Geometry: final body of the model. Coordinates: model frame, mm. A direction names the side the tool comes from. Round coordinates to 2 decimals unless told otherwise and drop trailing zeros. Loops run counter-clockwise (first coordinate to the right, second up) from the corner with the lowest first, then second, coordinate; pieces in that order, holes last. Notation, with made-up numbers: (-8.5, 80) - (37.5, 80) arc R8 cw to (37.5, 84) - close; hole circle Ø11 at (-35, -11.75). An arc over 180 degrees is marked (long way). Answer as CSV lines item,"result".
from build123d import *

# Parameters (mm, degrees)
SKETCH1_R           = 25.5
BOSS_EXTRUDE1_DEPTH = 4
SKETCH2_R           = 24.5
SKETCH2_R_2         = 18.5
CUT_EXTRUDE1_DEPTH  = 1.675
FILLET1_R           = 1.5
SKETCH3_R           = 14
CUT_EXTRUDE2_DEPTH  = 4
FILLET2_R           = 2
SKETCH4_R           = 1.25
CUT_EXTRUDE3_DEPTH  = 17
SKETCH5_R           = 1.25
CUT_EXTRUDE5_DEPTH  = 17


with BuildPart() as part:
    # Sketch1 → Boss-Extrude1 (new body)
    with BuildSketch(Plane.XY):
        Circle(SKETCH1_R)
    extrude(amount=BOSS_EXTRUDE1_DEPTH)

    # Sketch2 → Cut-Extrude1 (cut)
    with BuildSketch(Plane.XY.offset(4)):
        Circle(SKETCH2_R)
        Circle(SKETCH2_R_2, mode=Mode.SUBTRACT)
    extrude(amount=-CUT_EXTRUDE1_DEPTH, mode=Mode.SUBTRACT)

    # Fillet1
    fillet1_edges = [part.edges().sort_by_distance(p)[0] for p in [
        (-24.5, 0, 2.325),
        (-18.5, 0, 2.325),
    ]]
    fillet(fillet1_edges, radius=FILLET1_R)

    # Sketch3 → Cut-Extrude2 (cut)
    with BuildSketch(Plane.XY.offset(4)):
        Circle(SKETCH3_R)
    extrude(amount=-CUT_EXTRUDE2_DEPTH, mode=Mode.SUBTRACT)

    # Fillet2
    fillet2_edges = [part.edges().sort_by_distance(p)[0] for p in [
        (-25.5, 0, 0),
    ]]
    fillet(fillet2_edges, radius=FILLET2_R)

    # Sketch4 → Cut-Extrude3 (cut)
    with BuildSketch(Plane(origin=(0, 0, 0), x_dir=(0, 0, -1), z_dir=(1, 0, 0))):
        with Locations((-2, 0)):
            Circle(SKETCH4_R)
    extrude(amount=-CUT_EXTRUDE3_DEPTH, mode=Mode.SUBTRACT)

    # Sketch5 → Cut-Extrude5 (cut, symmetric)
    with BuildSketch(Plane(origin=(0, 0, 0), x_dir=(1, 0, 0), z_dir=(0, 1, 0))):
        with Locations(Location((-2.5, -2, 0), (0, 0, 270))):
            Circle(SKETCH5_R)
    extrude(amount=CUT_EXTRUDE5_DEPTH, both=True, mode=Mode.SUBTRACT)


solid = part.part
(1) Section B-B (x = 0). Output: boundary loops of the cut face in (y, z) (3 decimals).
Findings below:
outline,"(-25.5, 2) arc R2 ccw to (-23.5, 0) - (-14, 0) - (-14, 4) - (-18.5, 4) - (-18.5, 3.825) arc R1.5 cw to (-20, 2.325) - (-23, 2.325) arc R1.5 cw to (-24.5, 3.825) - (-24.5, 4) - (-25.5, 4) - close; (14, 0) - (23.5, 0) arc R2 ccw to (25.5, 2) - (25.5, 4) - (24.5, 4) - (24.5, 3.825) arc R1.5 cw to (23, 2.325) - (20, 2.325) arc R1.5 cw to (18.5, 3.825) - (18.5, 4) - (14, 4) - close"
(2) Draft query along Y for faces 1 (the face through (-3, 14, 4)), 2 (the face through (-5.5, -24.9, 3)), 3 (the face through (-2, -17, 2)). Return one class per face: pulls with the +Y half, pulls with the -Y half, needs draft (parallel to the pull), parting line crosses it, or undercut.
Findings below:
face 1,"needs draft"
face 2,"parting line crosses it"
face 3,"undercut"
(3) Section A-A (y = 0). Output: boundary loops of the cut face in (x, z) (3 decimals).
Findings below:
outline,"(-25.5, 2) arc R2 ccw to (-23.5, 0) - (-14, 0) - (-14, 0.75) - (-17, 0.75) - (-17, 3.25) - (-14, 3.25) - (-14, 4) - (-18.5, 4) - (-18.5, 3.825) arc R1.5 cw to (-20, 2.325) - (-23, 2.325) arc R1.5 cw to (-24.5, 3.825) - (-24.5, 4) - (-25.5, 4) - close; (14, 0) - (23.5, 0) arc R2 ccw to (25.5, 2) - (25.5, 4) - (24.5, 4) - (24.5, 3.825) arc R1.5 cw to (23, 2.325) - (20, 2.325) arc R1.5 cw to (18.5, 3.825) - (18.5, 4) - (14, 4) - close"
(4) Access query for faces 4 (the face through (-15.45, 0.38, 0.81)), 5 (the face through (-7, 19, 2.325)), 6 (the face through (13.35, 4.21, 2.03)). Directions: +Z, -Z, +X, -X, +Y, -Y. A direction counts if a zero-diameter tool reaches every point of the face in a straight line with its end or side. Return the directions, or none.
Findings below:
face 4,"none"
face 5,"+Z"
face 6,"+Z, -Z"
(5) Pin query (flat end, axial travel): P1, Ø1.5, axis at x = -2.5, z = 2, coming from the +Y side; P2, Ø1, axis at x = -1.5, z = 1.5, coming from the +Y side; P3, Ø2, axis at x = -2.5, z = 2, coming from the -Y side. Return the tip coordinate at first contact, or that it passes through.
Findings below:
P1,"y = 25.44"
P2,"y = 25.47"
P3,"y = -25.46"
(6) Material intervals for line 1 along Y through (x, z) = (0, 3.9); line 2 along Y through (x, z) = (16.5, 2.7); line 3 along X through (y, z) = (2.5, 2.6), sorted ascending.
Findings below:
line 1,"-25.5 to -24.5, -18.5 to -14, 14 to 18.5, 24.5 to 25.5"
line 2,"-19.44 to -17.42, -9.44 to 9.44, 17.42 to 19.44"
line 3,"-25.38 to -23.73, -18.97 to -13.77, 13.77 to 18.97, 23.73 to 25.38"
